```python
from build123d import *


with BuildPart() as part:
    # Esquisse1 → Révolution1 (revolve)
    with BuildSketch(Plane.XY, mode=Mode.PRIVATE) as r_volution1_sk:
        Polygon((28.95, 13), (28.95, 23.5), (43.95, 23.5), (43.95, 28.5), (-43.95, 28.5), (-43.95, 23.5), (-28.95, 23.5), (-28.95, 13), align=None)
    revolve(r_volution1_sk.sketch.rotate(Axis((-28.010573724, 0, 0), (1, 0, 0)), 90), axis=Axis((-28.010573724, 0, 0), (1, 0, 0)))  # turned: the seam where the file's is


solid = part.part
```
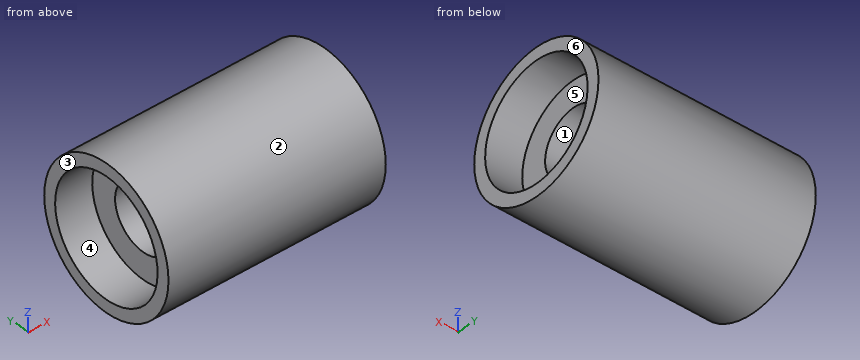
For this review, take the finished solid that the model builds, in its own axes (mm). Face numbers are marked on the shaded views. A direction names the side the tool comes from. Coordinates: 2 decimals unless noted, no trailing zeros. Order: outer loops, then holes, each group sorted by start corner. A loop starts at its lowest first (then second) coordinate and runs counter-clockwise, first axis right, second up. Notation, with made-up numbers: (33.5, 57.25) -> (60.5, 57.25) arc R24 cw to (60.5, 72.25) -> close; hole circle Ø1 at (-30, -22.75). An arc over 180 degrees is marked (long way). Use CSV: the item, a comma, the result in double quotes. Start each with the question number.
Item 1: We need section D-D, the plane x = 5.5. Give the boundary of the cut face in (y, z), then the cut area to 3 significant figures.
Item 2: We need section A-A, the plane z = 0. Give the boundary of the cut face in (x, y), then the cut area to 3 significant figures.
Item 3: For the marked faces 4, 5 and 6, list the 3-axis set-ups (+Z, -Z, +X, -X, +Y, -Y) from which the entire face can be reached by the end or side of a thin tool; tool diameter is ignored.
Item 4: Insertion check: pin 1 (6 mm diameter, centred on x = -22.5, z = -5.5, fed in from -Y); pin 2 (4 mm diameter, centred on x = -34.5, z = 9, fed in from +Y); pin 3 (3 mm diameter, centred on x = 6, z = -16, fed in from +Y); pin 4 (6 mm diameter, centred on y = -2.5, z = 7, fed in from +X). Each pin has a flat end and moves straight along its axis. Give the tip position at first contact, or say it passes through.
Item 5: Wall thickness on probe 1 along Y at (x, z) = (32, 0); probe 2 along X at (y, z) = (16.5, -13.5); probe 3 along Z at (x, y) = (5.5, -11): over which ranges is each line inside the solid? List them lowest first.
Item 6: We need section C-C, the plane x = -37. Give the boundary of the cut face in (y, z), then the cut area to 3 significant figures.
Item 7: Draft analysis for pull direction Z (two halves, no side actions). For the marked faces 1, 2 and 3, state which applies: pulls with the +Z half, pulls with the -Z half, needs draft (parallel to the pull), parting line crosses it, or undercut.
Derived:
1,outline,"circle Ø57 at (0, 0); hole circle Ø26 at (0, 0)"
1,area,"2,020 mm^2"
2,outline,"(-43.95, -28.5) -> (43.95, -28.5) -> (43.95, -23.5) -> (28.95, -23.5) -> (28.95, -13) -> (-28.95, -13) -> (-28.95, -23.5) -> (-43.95, -23.5) -> close; (-43.95, 23.5) -> (-28.95, 23.5) -> (-28.95, 13) -> (28.95, 13) -> (28.95, 23.5) -> (43.95, 23.5) -> (43.95, 28.5) -> (-43.95, 28.5) -> close"
2,area,"2,090 mm^2"
3,face 4,"-X"
3,face 5,"+X"
3,face 6,"+Z, -Z, +X, +Y, -Y"
4,pin 1,"stops at y = -28.39"
4,pin 2,"stops at y = 27.63"
4,pin 3,"stops at y = 24.54"
4,pin 4,"passes through"
5,probe 1,"y = -28.5 to -23.5, 23.5 to 28.5"
5,probe 2,"x = -28.95 to 28.95"
5,probe 3,"z = -26.29 to -6.93, 6.93 to 26.29"
6,outline,"circle Ø57 at (0, 0); hole circle Ø47 at (0, 0)"
6,area,"817 mm^2"
7,face 1,"undercut"
7,face 2,"parting line crosses it"
7,face 3,"needs draft"
